Design review of the part built by this model. Coordinates are the model's own, in mm. Coordinates: 2 decimals unless noted, no trailing zeros. Loops run counter-clockwise (first coordinate to the right, second up) from the corner with the lowest first, then second, coordinate; pieces in that order, holes last. Notation, with made-up numbers: (51, 36) - (105, 36) arc R26 cw to (105, 50) - close; hole circle Ø7 at (80.5, 48). An arc over 180 degrees is marked (long way). One line per question, with ' | ' between items.
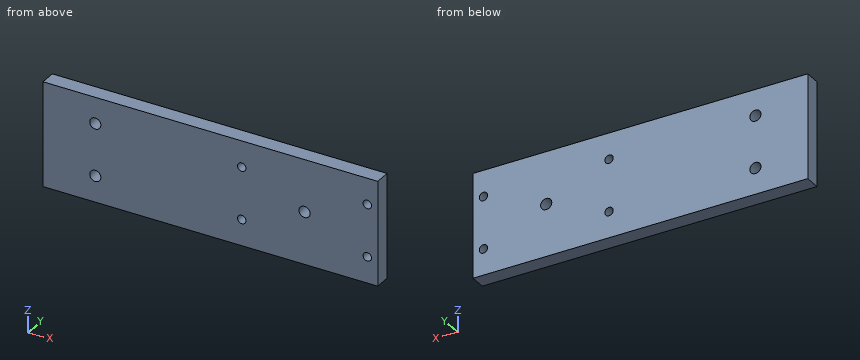
from build123d import *

# Parameters (mm, degrees)
SKETCH1_W               = 203.2
SKETCH1_H               = 63.5
BOSS_EXTRUDE1_DEPTH     = 9.525
F_10_CLEARANCE_HOLE1_D  = 5.1054
F_1_4_CLEARANCE_HOLE1_D = 6.7564
F_1_4_CLEARANCE_HOLE2_D = 6.7564


with BuildPart() as part:
    # Sketch1 → Boss-Extrude1 (new body)
    with BuildSketch(Plane(origin=(0, 0, 0), x_dir=(1, 0, 0), z_dir=(0, 1, 0))):
        Rectangle(SKETCH1_W, SKETCH1_H)
    extrude(amount=BOSS_EXTRUDE1_DEPTH)

    # #10 Clearance Hole1 (through all)
    with Locations(Plane(origin=(0, 0, 0), x_dir=(-1, 0, 0), z_dir=(0, -1, 0))):
        with Locations((-19.05, 15.875), (-95.25, 15.875), (-95.25, -15.875), (-19.05, -15.875)):
            Hole(F_10_CLEARANCE_HOLE1_D / 2)

    # 1/4 Clearance Hole1 (through all)
    with Locations(Plane(origin=(0, 0, 0), x_dir=(-1, 0, 0), z_dir=(0, -1, 0))):
        with Locations((-57.15, 0)):
            Hole(F_1_4_CLEARANCE_HOLE1_D / 2)

    # 1/4 Clearance Hole2 (through all)
    with Locations(Plane(origin=(0, 0, 0), x_dir=(-1, 0, 0), z_dir=(0, -1, 0))):
        with Locations((69.85, 15.875), (69.85, -15.875)):
            Hole(F_1_4_CLEARANCE_HOLE2_D / 2)


solid = part.part
Q1. Take a section at C-C (z = 0). Give the boundary of the cut face in (x, y) (3 decimals), plus the area to 3 significant figures.
Returned:
outline: (-101.6, 0) - (53.772, 0) - (53.772, 9.525) - (-101.6, 9.525) - close; (60.528, 0) - (101.6, 0) - (101.6, 9.525) - (60.528, 9.525) - close | area: 1,870 mm²
Q2. Take a section at B-B (x = 19.05). Give the boundary of the cut face in (y, z) (3 decimals), plus the area to 3 significant figures.
Returned:
outline: (0, -31.75) - (9.525, -31.75) - (9.525, -18.428) - (0, -18.428) - close; (0, -13.322) - (9.525, -13.322) - (9.525, 13.322) - (0, 13.322) - close; (0, 18.428) - (9.525, 18.428) - (9.525, 31.75) - (0, 31.75) - close | area: 508 mm²
Q3. Take a section at D-D (x = -69.85). Give the boundary of the cut face in (y, z) (3 decimals).
Returned:
outline: (0, -31.75) - (9.525, -31.75) - (9.525, -19.253) - (0, -19.253) - close; (0, -12.497) - (9.525, -12.497) - (9.525, 12.497) - (0, 12.497) - close; (0, 19.253) - (9.525, 19.253) - (9.525, 31.75) - (0, 31.75) - close
Q4. To check wall thickness, follow line 1 along Z through (x, y) = (-70, 2.5); line 2 along Z through (x, y) = (95.25, 5.75); line 3 along X through (y, z) = (4.75, 14.5). State the ranges of each line that lie inside material, in increasing order.
Returned:
line 1: z = -31.75 to -19.25, -12.5 to 12.5, 19.25 to 31.75 | line 2: z = -31.75 to -18.43, -13.32 to 13.32, 18.43 to 31.75 | line 3: x = -101.6 to -72.94, -66.76 to 16.9, 21.2 to 93.1, 97.4 to 101.6
Q5. Take a section at A-A (x = 57.15). Give the boundary of the cut face in (y, z) (3 decimals), plus the area to 3 significant figures.
Returned:
outline: (0, -31.75) - (9.525, -31.75) - (9.525, -3.378) - (0, -3.378) - close; (0, 3.378) - (9.525, 3.378) - (9.525, 31.75) - (0, 31.75) - close | area: 540 mm²
